Part print with two shaded views. Sizes in mm from the minimum x, y, z corner. A direction names the side the tool comes from. Give positions to 0.01 mm unless a question says otherwise; leave off trailing zeros. Write each loop counter-clockwise with the first axis right and the second up, starting at its lowest first coordinate (ties: lowest second). Pieces come first, ordered by that corner, then holes.
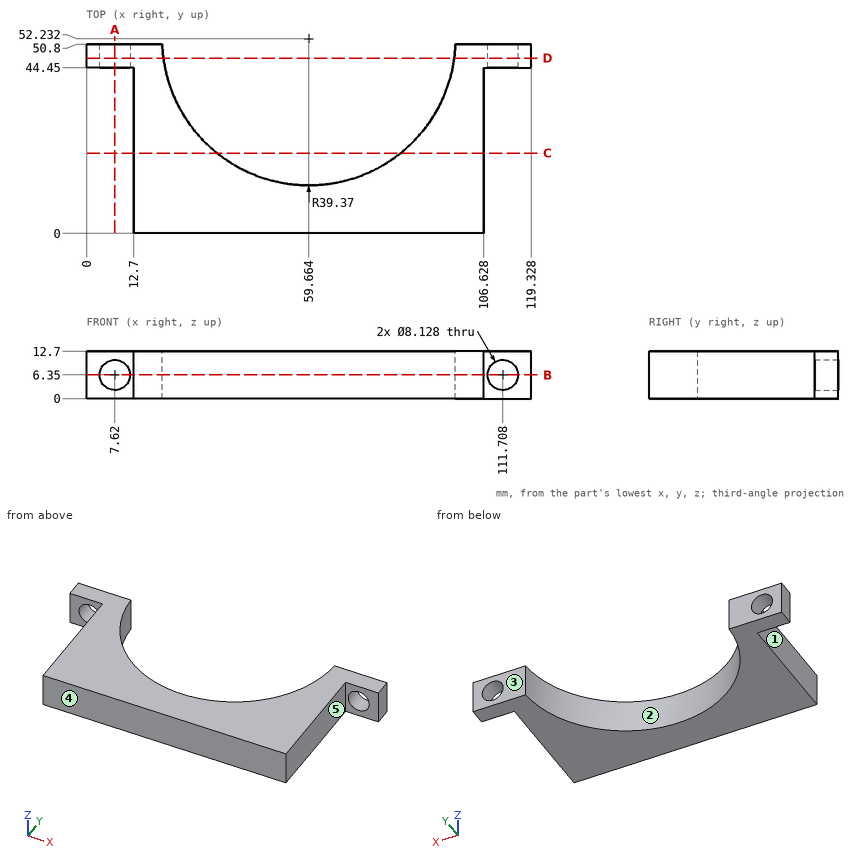
1) Saw through at B-B, the plane z = 6.35. Write the cut outline in (x, y).
Answers follow:
outline: (0, 44.45) - (3.56, 44.45) - (3.56, 50.8) - (0, 50.8) - close; (11.68, 44.45) - (12.7, 44.45) - (12.7, 0) - (106.63, 0) - (106.63, 44.45) - (107.64, 44.45) - (107.64, 50.8) - (99.01, 50.8) arc R39.37 cw to (20.32, 50.8) - (11.68, 50.8) - close; (115.77, 44.45) - (119.33, 44.45) - (119.33, 50.8) - (115.77, 50.8) - close
2) Two-plate mould, pull along X, no slides. Class the marked faces 1, 2 and 3: +X half, -X half, draft (parallel to the pull), parting line (faces both ways), or undercut.
Answers follow:
face 1: -X half
face 2: undercut
face 3: draft
3) 3-axis set-ups, long thin cutter, end or side, ignore diameter. For the marked faces 4 and 5: which of +Z, -Z, +X, -X, +Y, -Y reach the whole face in a straight line?
Answers follow:
face 4: +Z, -Z, +X, -X, -Y
face 5: +Z, -Z, +X, -Y
4) Wall check: L1, parallel to X at y = 47.25, z = 6.35 (1 decimal); L2, parallel to X at y = 48.25, z = 6.35 (1 decimal); L3, parallel to Z at x = 7.62, y = 48. Give the ranges that are in metal, low to high.
Answers follow:
L1: x = 0 to 3.6, 11.7 to 20.6, 98.7 to 107.6, 115.8 to 119.3
L2: x = 0 to 3.6, 11.7 to 20.5, 98.8 to 107.6, 115.8 to 119.3
L3: z = 0 to 2.29, 10.41 to 12.7
5) Saw through at A-A, the plane x = 7.62. Write the cut outline in (y, z).
Answers follow:
outline: (44.45, 0) - (50.8, 0) - (50.8, 2.29) - (44.45, 2.29) - close; (44.45, 10.41) - (50.8, 10.41) - (50.8, 12.7) - (44.45, 12.7) - close
6) Pin check, flat tips, straight feed: pin 1 Ø6.5 at (x, z) = (114, 4.5) entering from -Y; pin 2 Ø4 at (y, z) = (21.5, 8) entering from -X; pin 3 Ø5 at (y, z) = (19.5, 6) entering from +X. Stop position of each tip, or through.
Answers follow:
pin 1: stops at y = 44.45
pin 2: stops at x = 12.7
pin 3: stops at x = 106.63
7) Saw through at C-C, the plane y = 21.5. Write the cut outline in (x, z) (1 decimal).
Answers follow:
outline: (12.7, 0) - (35.1, 0) - (35.1, 12.7) - (12.7, 12.7) - close; (84.3, 0) - (106.6, 0) - (106.6, 12.7) - (84.3, 12.7) - close
8) Saw through at D-D, the plane y = 47. Count the separate pieces of the cut face and the enclosed holes in it.
Answers follow:
separate pieces: 2
enclosed holes: 2
